Geometry check sheet. Reference: drawing and pictorial views, mm from the part's lowest x, y, z. A direction names the side the tool comes from. Coordinates: 2 decimals unless noted, no trailing zeros. Loops run counter-clockwise (first coordinate to the right, second up) from the corner with the lowest first, then second, coordinate; pieces in that order, holes last. Notation, with made-up numbers: (-18.5, 45.5) -> (38.5, 45.5) arc R33 ccw to (38.5, 75.5) -> close; hole circle Ø2 at (-33.75, -22). An arc over 180 degrees is marked (long way). Answer as a JSON object with one key per item and string values. Group by question number.
Q1. Gauge pin test, flat ends, axial feed: pin 1 Ø6 at (y, z) = (4.5, 9.5) entering from -X; pin 2 Ø3.5 at (x, z) = (5.5, 5.5) entering from +Y; pin 3 Ø1 at (y, z) = (9, 10) entering from -X. Record the tip position at first contact, or that the pin passes through.
Q2. Set-up check for the marked faces 4, 5, 6 and 7: record each of +Z, -Z, +X, -X, +Y, -Y from which the full face is reachable in a straight line by a thin tool's end or side.
Q3. Cross-section at D-D on z = 3. Record the boundary of the cut face in (x, y), and give its area (3 significant figures).
Q4. Cross-section at B-B on x = 5.5. Record the boundary of the cut face in (y, z), and give its area (3 significant figures).
Q5. Scan lines: L1, parallel to Y at x = 10.5, z = 6.75; L2, parallel to Z at x = 5.5, y = 13.75. Record each from-to range of solid material in increasing order.
Q6. Release check for a two-part mould opening along X. For the marked faces 1, 2 and 3 record: released by +X, released by -X, zero draft, split by the parting line, or undercut.
Q7. Cross-section at A-A on z = 10.25. Record the boundary of the cut face in (x, y), and give its area (3 significant figures).
Q8. Cross-section at C-C on y = 1.75. Record the boundary of the cut face in (x, z).
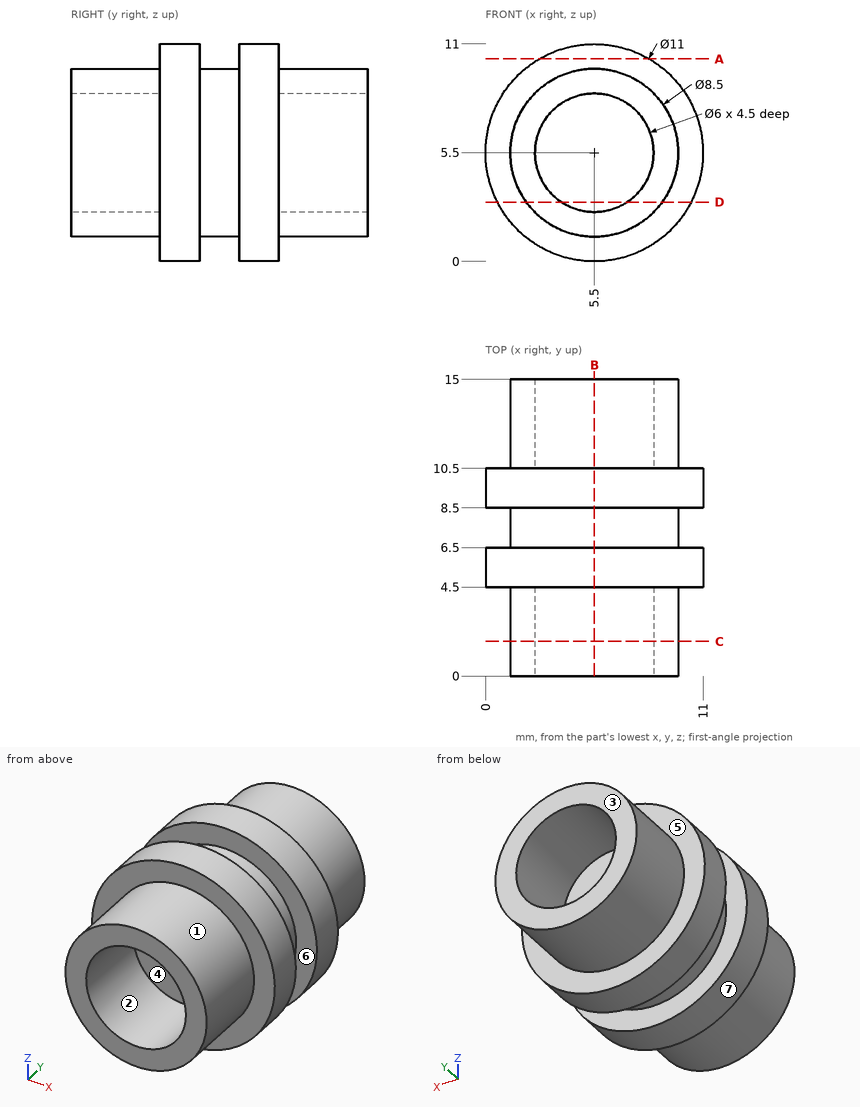
Computed values:
{
 "1": {"pin 1": "stops at x = 0.09", "pin 2": "stops at y = 10.5", "pin 3": "stops at x = 1.73"},
 "2": {"face 4": "-Y", "face 5": "+Y", "face 6": "none", "face 7": "+Y, -Y"},
 "3": {"outline": "(0.6, 4.5) -> (2.06, 4.5) -> (2.06, 0) -> (3.84, 0) -> (3.84, 4.5) -> (7.16, 4.5) -> (7.16, 0) -> (8.94, 0) -> (8.94, 4.5) -> (10.4, 4.5) -> (10.4, 6.5) -> (8.94, 6.5) -> (8.94, 8.5) -> (10.4, 8.5) -> (10.4, 10.5) -> (8.94, 10.5) -> (8.94, 15) -> (7.16, 15) -> (7.16, 10.5) -> (3.84, 10.5) -> (3.84, 15) -> (2.06, 15) -> (2.06, 10.5) -> (0.6, 10.5) -> (0.6, 8.5) -> (2.06, 8.5) -> (2.06, 6.5) -> (0.6, 6.5) -> close", "area": "85.0 mm²"},
 "4": {"outline": "(0, 1.25) -> (4.5, 1.25) -> (4.5, 0) -> (6.5, 0) -> (6.5, 1.25) -> (8.5, 1.25) -> (8.5, 0) -> (10.5, 0) -> (10.5, 1.25) -> (15, 1.25) -> (15, 2.5) -> (10.5, 2.5) -> (10.5, 8.5) -> (15, 8.5) -> (15, 9.75) -> (10.5, 9.75) -> (10.5, 11) -> (8.5, 11) -> (8.5, 9.75) -> (6.5, 9.75) -> (6.5, 11) -> (4.5, 11) -> (4.5, 9.75) -> (0, 9.75) -> (0, 8.5) -> (4.5, 8.5) -> (4.5, 2.5) -> (0, 2.5) -> close", "area": "83.5 mm²"},
 "5": {"L1": "y = 4.5 to 6.5, 8.5 to 10.5", "L2": "z = 1.25 to 2.5, 8.5 to 9.75"},
 "6": {"face 1": "split by the parting line", "face 2": "undercut", "face 3": "zero draft"},
 "7": {"outline": "(2.73, 4.5) -> (8.27, 4.5) -> (8.27, 6.5) -> (2.73, 6.5) -> close; (2.73, 8.5) -> (8.27, 8.5) -> (8.27, 10.5) -> (2.73, 10.5) -> close", "area": "22.2 mm²"},
 "8": {"outline": "circle Ø8.5 at (5.5, 5.5); hole circle Ø6 at (5.5, 5.5)"}
}
